Source: CAD feature listing. Evaluate the final solid. Frame: model axes, mm. A direction names the side the tool comes from. Coordinates: 2 decimals unless noted, no trailing zeros. Loops run counter-clockwise (first coordinate to the right, second up) from the corner with the lowest first, then second, coordinate; pieces in that order, holes last.
Item 1: Reachability of faces 1 (the cylindrical face through (1.63, -133.32, -8.54)), 2 (the flat face through (0, -126, -20)) from +Z, -Z, +X, -X, +Y, -Y: full face, straight path, thin tool, end or side. Return the list, or none.
Item 2: Section query A-A, the plane y = -121.5. Return the cut outline in (x, z), then the cut area to 3 significant figures.
Item 3: Section query D-D, the plane y = -86. Return the cut outline in (x, z), then the cut area to 3 significant figures.
Item 4: Section query C-C, the plane z = 5. Return the cut outline in (x, y).
Item 5: Pin query (flat end, axial travel): pin 1 Ø5 at (y, z) = (-74.5, -1) entering from +X; pin 2 Ø1.5 at (x, z) = (-5.5, 4) entering from -Y; pin 3 Ø2 at (x, z) = (2.5, 21) entering from +Y; pin 4 Ø1.5 at (x, z) = (4, 15) entering from +Y. Return the tip coordinate at first contact, or that it passes through.
Item 6: Line query: probe 1 along Z at (x, y) = (-3.5, -69.5); probe 2 along Z at (x, y) = (-5.5, -2); probe 3 along Y at (x, z) = (1.25, -2.5). Output: solid intervals per line, ascending.
Item 7: Section query B-B, the plane x = 0. Return the cut outline in (y, z), then the cut area to 3 significant figures.
```python
from build123d import *

# Parameters (mm, degrees)
EXTRUDE_1_DEPTH = 10
SKETCH_2_R      = 7.5
EXTRUDE_2_DEPTH = 20
EXTRUDE_START   = 20
SKETCH_3_R      = 7.5
EXTRUDE_3_DEPTH = 20


with BuildPart() as part:
    # 草图1 → 凸台-拉伸1 (new body)
    with BuildSketch(Plane.XY):
        with BuildLine():
            Line((7.5, 0), (7.5, -126))
            ThreePointArc((7.5, -126), (0, -133.5), (-7.5, -126))
            Line((-7.5, -126), (-7.5, 0))
            ThreePointArc((-7.5, 0), (0, 7.5), (7.5, 0))
        make_face()
    extrude(amount=EXTRUDE_1_DEPTH)

    # 草图2 → 凸台-拉伸2 (add)
    with BuildSketch(Plane.XY.offset(10)):
        Circle(SKETCH_2_R)
    extrude(amount=EXTRUDE_2_DEPTH)

    # 草图3 → 凸台-拉伸3 (add)
    with BuildSketch(Plane(origin=(0, 0, 0), x_dir=(-1, 0, 0), z_dir=(0, 0, -1)).offset(EXTRUDE_START)):
        with Locations((0, -126)):
            Circle(SKETCH_3_R)
    extrude(amount=-EXTRUDE_3_DEPTH)


solid = part.part
```
Verdict:
1. face 1: -Z
1. face 2: -Z, +X, -X, +Y, -Y
2. outline: (-7.5, 0) - (-6, 0) - (-6, -20) - (6, -20) - (6, 0) - (7.5, 0) - (7.5, 10) - (-7.5, 10) - close
2. area: 390 mm2
3. outline: (-7.5, 0) - (7.5, 0) - (7.5, 10) - (-7.5, 10) - close
3. area: 150 mm2
4. outline: (-7.5, -126) arc R7.5 ccw to (7.5, -126) - (7.5, 0) arc R7.5 ccw to (-7.5, 0) - close
5. pin 1: stops at x = 7.5
5. pin 2: stops at y = -131.8
5. pin 3: stops at y = 7.35
5. pin 4: stops at y = 6.76
6. probe 1: z = 0 to 10
6. probe 2: z = 0 to 30
6. probe 3: y = -133.4 to -118.6
7. outline: (-133.5, -20) - (-118.5, -20) - (-118.5, 0) - (7.5, 0) - (7.5, 30) - (-7.5, 30) - (-7.5, 10) - (-133.5, 10) - close
7. area: 2,010 mm2
